```python
from build123d import *

# Parameters (mm, degrees)
SALIENTE_EXTRUIR1_DEPTH = 7.9375
CROQUIS4_R              = 3.75
SALIENTE_EXTRUIR5_DEPTH = 3.175
CORTAR_EXTRUIR2_DEPTH   = 7.9375
CORTAR_EXTRUIR1_DEPTH   = 1.7145


with BuildPart() as part:
    # Croquis1 → Saliente-Extruir1 (new body)
    with BuildSketch(Plane.XY):
        with BuildLine():
            Line((9.02, -8.199999983), (9.02, -4.401948997))
            ThreePointArc((9.02, -4.401948997), (0, 10.03681), (-9.02, -4.401948997))
            Line((-9.02, -4.401948997), (-9.02, -8.465948997))
            Line((-9.02, -8.465948997), (-9.02, -16.593948997))
            Line((-9.02, -16.593948997), (-7.75, -16.593948997))
            Line((-7.75, -16.593948997), (-7.75, -8.465948997))
            Line((-7.75, -8.465948997), (-7.75, -3.365759866))
            ThreePointArc((-7.75, -3.365759866), (0, 8.44931), (7.75, -3.365759866))
            Line((7.75, -3.365759866), (7.75, -8.199999983))
            Line((7.75, -8.199999983), (7.75, -16.593948997))
            Line((7.75, -16.593948997), (9.02, -16.593948997))
            Line((9.02, -16.593948997), (9.02, -8.199999983))
        make_face()
    extrude(amount=SALIENTE_EXTRUIR1_DEPTH)

    # Croquis4 → Saliente-Extruir5 (add)
    with BuildSketch(Plane.XY):
        with BuildLine():
            Line((-11.302677464, -5.515943429), (-11.302677464, -16.593948997))
            Line((-11.302677464, -16.593948997), (-9.02, -16.593948997))
            Line((-9.02, -16.593948997), (9.02, -16.593948997))
            Line((9.02, -16.593948997), (11.302677464, -16.593948997))
            Line((11.302677464, -16.593948997), (11.302677464, -5.515943429))
            ThreePointArc((11.302677464, -5.515943429), (0, 12.57681), (-11.302677464, -5.515943429))
        make_face()
        Circle(CROQUIS4_R, mode=Mode.SUBTRACT)
    extrude(amount=-SALIENTE_EXTRUIR5_DEPTH)

    # Croquis6 → Cortar-Extruir2 (cut)
    with BuildSketch(Plane.XY.offset(7.9375)):
        with BuildLine():
            Line((-8.041222005, -3.492235135), (-7.75, -3.365759866))
            ThreePointArc((-7.75, -3.365759866), (-8.145389049, 2.245768624), (-4.930152432, 6.86181))
            Line((-4.930152432, 6.86181), (-5.115412932, 7.11965646))
            ThreePointArc((-5.115412932, 7.11965646), (-8.451468602, 2.330157945), (-8.041222005, -3.492235135))
        make_face()
        with BuildLine():
            Line((7.75, -3.365759866), (8.048475458, -3.474012585))
            ThreePointArc((8.048475458, -3.474012585), (8.275668302, 2.281687971), (5.130979952, 7.107725752))
            Line((5.130979952, 7.107725752), (4.930152432, 6.86181))
            ThreePointArc((4.930152432, 6.86181), (7.96958875, 2.19729865), (7.75, -3.365759866))
        make_face()
    extrude(amount=-CORTAR_EXTRUIR2_DEPTH, mode=Mode.SUBTRACT)

    # Croquis5 → Cortar-Extruir1 (cut)
    with BuildSketch(Plane.XY):
        with BuildLine():
            Line((6.854573627, -3.041001708), (8.048475458, -3.474012585))
            ThreePointArc((8.048475458, -3.474012585), (8.609503442, -0.613823624), (8.275668302, 2.281687971))
            Line((8.275668302, 2.281687971), (7.051350093, 1.944130685))
            ThreePointArc((7.051350093, 1.944130685), (7.340491675, -0.563732346), (6.854573627, -3.041001708))
        make_face()
    extrude(amount=-CORTAR_EXTRUIR1_DEPTH, mode=Mode.SUBTRACT)


solid = part.part
```
Model file for the job. Use its own axes, mm. A direction names the side the tool comes from. Coordinates: 2 decimals unless noted, no trailing zeros. Order: outer loops, then holes, each group sorted by start corner. A loop starts at its lowest first (then second) coordinate and runs counter-clockwise, first axis right, second up. Notation, with made-up numbers: (13, 87) -> (49, 87) arc R31 ccw to (49, 120) -> close; hole circle Ø10 at (45.25, -4). An arc over 180 degrees is marked (long way). Answer as a JSON object with one key per item and string values. Group by question number.
1) Flat gauge pins, fed straight in: pin 1 (2.5 mm diameter, centred on y = -11, z = 4.5, fed in from -X); pin 2 (3.5 mm diameter, centred on y = -11, z = -1.5, fed in from -X); pin 3 (6.5 mm diameter, centred on y = -7.5, z = 4.5, fed in from +X); pin 4 (7 mm diameter, centred on x = 0, y = 0, fed in from -Z). Where does each tip first touch, or does it go through?
2) Cut at C-C, the plane y = -2. Write the cut outline in (x, z) (1 decimal), then the cut area to 3 significant figures.
3) Cut at D-D, the plane z = 1.5. Write the cut outline in (x, y).
4) Cut at B-B, the plane z = -0.5. Write the cut outline in (x, y), then the cut area to 3 significant figures.
5) Drill centre lines: L1, parallel to X at y = -4.5, z = 3; L2, parallel to X at y = 0, z = 2.75; L3, parallel to Y at x = 0, z = -1.1. Where is each one in solid material? Low to high.
6) Which spindle directions (+Z, -Z, +X, -X, +Y, -Y) get a long thin tool onto all of the face, cutting with end or side? Do faces 1 (the face through (-11.303, -11, -2)), 2 (the face through (7.34, -0.53, -0.85)), 3 (the face through (-9.02, -10, 4)). Say none if no direction does.
7) Pull direction X, two halves, no side cores. Call faces 4 (the face through (11.303, -11, -2)), 5 (the face through (7.75, -10, 4)), 6 (the face through (-10.3, -0.9, 0)): +X half, -X half, draft (parallel to the pull), parting line (faces both ways), or undercut.
Check values:
{
 "1": {"pin 1": "stops at x = -9.02", "pin 2": "stops at x = -11.3", "pin 3": "stops at x = 9.09", "pin 4": "passes through"},
 "2": {"outline": "(-12.4, -3.2) -> (-3.2, -3.2) -> (-3.2, 0) -> (-8.5, 0) -> (-8.5, 7.9) -> (-9.8, 7.9) -> (-9.8, 0) -> (-12.4, 0) -> close; (3.2, -3.2) -> (12.4, -3.2) -> (12.4, 0) -> (9.8, 0) -> (9.8, 7.9) -> (8.5, 7.9) -> (8.5, -1.7) -> (7.2, -1.7) -> (7.2, 0) -> (3.2, 0) -> close", "area": "77.8 mm²"},
 "3": {"outline": "(-9.02, -16.59) -> (-7.75, -16.59) -> (-7.75, -3.37) -> (-8.04, -3.49) arc R8.77 cw to (-5.12, 7.12) -> (-4.93, 6.86) arc R8.45 cw to (4.93, 6.86) -> (5.13, 7.11) arc R9.49 cw to (8.05, -3.47) -> (7.75, -3.37) -> (7.75, -16.59) -> (9.02, -16.59) -> (9.02, -4.4) arc R10.04 ccw (long way) to (-9.02, -4.4) -> close"},
 "4": {"outline": "(-11.3, -16.59) -> (11.3, -16.59) -> (11.3, -5.52) arc R12.58 ccw (long way) to (-11.3, -5.52) -> close; hole circle Ø7.5 at (0, 0); hole (6.85, -3.04) -> (8.05, -3.47) arc R9.49 ccw to (8.28, 2.28) -> (7.05, 1.94) arc R8.22 cw to start", "area": "582 mm²"},
 "5": {"L1": "x = -9.02 to -7.75, 7.75 to 9.02", "L2": "x = -10.04 to -8.77, 8.61 to 10.04", "L3": "y = -16.59 to -3.75, 3.75 to 12.58"},
 "6": {"face 1": "+Z, -Z, -X, -Y", "face 2": "+Z", "face 3": "+Z, -X, -Y"},
 "7": {"face 4": "+X half", "face 5": "undercut", "face 6": "draft"}
}
